Read the model definition and answer for the solid it produces. Units are mm, in the model's axes. A direction names the side the tool comes from. Give positions to 0.01 mm unless a question says otherwise; leave off trailing zeros. Write each loop counter-clockwise with the first axis right and the second up, starting at its lowest first coordinate (ties: lowest second). Pieces come first, ordered by that corner, then holes.
```python
from build123d import *

# Parameters (mm, degrees)
F0_R     = 8.25
F0_R_2   = 3
F1_DEPTH = 1.5
F2_R     = 8.25
F2_R_2   = 7
F3_DEPTH = 31
F4_R     = 7.75
F4_R_2   = 7
F5_DEPTH = 2
F7_ANGLE = 90


with BuildPart() as f1:
    # F0 (on Top) → F1 (new body)
    with BuildSketch(Plane.XY):
        Circle(F0_R)
        Circle(F0_R_2, mode=Mode.SUBTRACT)
    extrude(amount=F1_DEPTH)

    # F2 (on face) → F3 (join)
    with BuildSketch(Plane.XY.offset(1.5)):
        Circle(F2_R)
        Circle(F2_R_2, mode=Mode.SUBTRACT)
    extrude(amount=F3_DEPTH)

    # F4 (on face) → F5 (join)
    with BuildSketch(Plane.XY.offset(32.5)):
        Circle(F4_R)
        Circle(F4_R_2, mode=Mode.SUBTRACT)
    extrude(amount=F5_DEPTH)


with BuildPart() as f1_1:
    # F7: moved
    add(f1.part.rotate(Axis((6.326988, 0, 0), (1, 0, 0)), F7_ANGLE))


solid = f1_1.part
```
Item 1: Section D-D (z = -6.5) is taken. Write down the section's boundary in (x, y), and give its area (3 significant figures).
Result set:
outline: (-5.08, -32.5) - (-4.22, -32.5) - (-4.22, -34.5) - (-2.6, -34.5) - (-2.6, -1.5) - (2.6, -1.5) - (2.6, -34.5) - (4.22, -34.5) - (4.22, -32.5) - (5.08, -32.5) - (5.08, 0) - (-5.08, 0) - close
area: 176 mm2
Item 2: Each of these flat-tipped pins is pushed along its axis until it touches: pin 1 Ø5 at (y, z) = (-13.5, 1.5) entering from -X; pin 2 Ø3 at (y, z) = (-12.5, -3.5) entering from -X; pin 3 Ø2 at (x, y) = (5, -14) entering from -Z; pin 4 Ø4 at (x, z) = (3, 2.5) entering from -Y. Where does it stop, or does it pass through?
Result set:
pin 1: stops at x = -8.25
pin 2: stops at x = -8
pin 3: stops at z = -7.22
pin 4: stops at y = -1.5
Item 3: Section A-A (x = 0) is taken. Write down the section's boundary in (y, z), and give its area (4 significant figures).
Result set:
outline: (-34.5, -7.75) - (-32.5, -7.75) - (-32.5, -8.25) - (0, -8.25) - (0, -3) - (-1.5, -3) - (-1.5, -7) - (-34.5, -7) - close; (-34.5, 7) - (-1.5, 7) - (-1.5, 3) - (0, 3) - (0, 8.25) - (-32.5, 8.25) - (-32.5, 7.75) - (-34.5, 7.75) - close
area: 96.25 mm2
Item 4: Which of the six approach directions +Z, -Z, +X, -X, +Y, -Y give full straight-line access (tool end or side, diameter ignored) to faces 1 (the cylindrical face through (6.466, -17.769, -2.681)), 2 (the flat face through (0, 0, -4))?
Result set:
face 1: -Y
face 2: +Z, -Z, +X, -X, +Y
Item 5: Determine the mould class of faces 3 (the flat face through (-6, -34.5, -4)), 4 (the cylindrical face through (-1.788, -16.022, -8.054)), 5 (the cylindrical face through (-3, -1, 0)) for opening direction X: pulls with the +X half, pulls with the -X half, needs draft (parallel to the pull), parting line crosses it, or undercut.
Result set:
face 3: needs draft
face 4: parting line crosses it
face 5: undercut
Item 6: Section B-B (z = 0) is taken. Write down the section's boundary in (x, y).
Result set:
outline: (-8.25, -32.5) - (-7.75, -32.5) - (-7.75, -34.5) - (-7, -34.5) - (-7, -1.5) - (-3, -1.5) - (-3, 0) - (-8.25, 0) - close; (3, -1.5) - (7, -1.5) - (7, -34.5) - (7.75, -34.5) - (7.75, -32.5) - (8.25, -32.5) - (8.25, 0) - (3, 0) - close
Item 7: Section C-C (y = -10) is taken. Write down the section's boundary in (x, z).
Result set:
outline: circle Ø16.5 at (0, 0); hole circle Ø14 at (0, 0)
Item 8: Find the intervals of material crossed by line 1 along Z through (x, y) = (0, -14.5); line 2 along Z through (x, y) = (0, -1); line 3 along X through (y, z) = (-13.5, 5.5), in increasing order.
Result set:
line 1: z = -8.25 to -7, 7 to 8.25
line 2: z = -8.25 to -3, 3 to 8.25
line 3: x = -6.15 to -4.33, 4.33 to 6.15
